Geometry: final body of the model. Coordinates: model frame, mm. A direction names the side the tool comes from. Round coordinates to 2 decimals unless told otherwise and drop trailing zeros. Order: outer loops, then holes, each group sorted by start corner. A loop starts at its lowest first (then second) coordinate and runs counter-clockwise, first axis right, second up. Notation, with made-up numbers: M -15,15 L 22,15 A25 cw 22,38 Z; hole C 71,34 d1. An arc over 180 degrees is marked long. Put each result on its own line as item: value. Start each with the question number.
1) Section D-D, the plane x = 3.5. Return loops of the section in (y, z), then the cut area to 3 significant figures.
2) Section B-B, the plane z = 0. Return loops of the section in (x, y), then the cut area to 3 significant figures.
3) Access query for faces 1 (the flat face through (-6.467, 15.21, 4.441)), 2 (the flat face through (6, 15, -10.95)), 3 (the flat face through (0, 15, -9)), 4 (the flat face through (9.5, 8, 0)), 5 (the cylindrical face through (-2.62, 14.79, 5.34)). Directions: +Z, -Z, +X, -X, +Y, -Y. A direction counts if a zero-diameter tool reaches every point of the face in a straight line with its end or side. Return the directions, or none.
4) Section A-A, the plane x = -2.5. Return loops of the section in (y, z), then the cut area to 3 significant figures.
5) First-contact query: P1, Ø3, axis at x = -4.5, y = 19.5, coming from the -Z side; P2, Ø9, axis at y = 22, z = 0, coming from the +X side; P3, Ø3, axis at x = -2, y = 21.5, coming from the -Z side. Flat tips, straight axial feed; report the tip coordinate or a pass-through.
6) Material intervals for probe 1 along Y at (x, z) = (10.4, 0); probe 2 along Z at (x, y) = (10.85, 8); probe 3 along X at (y, z) = (25.25, 4.5), sorted ascending. Write a range as [from, to].
7) Draft query along Z for faces 6 (the flat face through (0, 15, 9)), 7 (the flat face through (-6.467, 15.21, -4.441)), 8 (the cylindrical face through (-2.7, 14.8, -5.3)). Return one class per face: pulls with the +Z half, pulls with the -Z half, needs draft (parallel to the pull), parting line crosses it, or undercut.
Autodesk Inventor part; units mm, degrees
ref_plane "YZ Plane" through (0, 0, 0) normal (1, 0, 0) x (0, 1, 0)
ref_plane "XZ Plane" through (0, 0, 0) normal (0, 1, 0) x (-1, 0, 0)
ref_plane "XY Plane" through (0, 0, 0) normal (0, 0, 1) x (1, 0, 0)
sketch "Эскиз1" plane through (0, 0, 0) normal (0, 1, 0) x (-1, 0, 0)
  circle A0 centre (0, 0) radius 5.95
  circle A1 centre (0, 0) radius 6.95
  line L0 (0, 0) -> (5.546, 4.1887)
  line L1 (0, 0) -> (5.546, -4.1887)
  point P0 (4.748, -3.586)
  point P1 (4.748, 3.586)
  dimension "d0" = 11.9
  dimension "d1" = 13.9
extrude "Выдавливание1" add sketch "Эскиз1" along normal blind 30 contours A0 L1 A1 L0 picked at (4.878, 4.401)
sketch "Эскиз2" plane through (0, 30, 0) normal (0, 1, 0) x (1, 0, 0)
  arc A0 (-4.748, -3.586) -> (-5.6407, -3.0561) centre (-7.4493, -7.1199) ccw
  arc A1 (-5.6407, -3.0561) -> (-6.7976, -4.8618) centre (-6.075, -4.0513) ccw
  line L0 (-6.7976, -4.8618) -> (-6.1263, -4.0074)
  arc A2 (-5.5474, -4.1741) -> (-6.1263, -4.0074) centre (-5.9157, -4.3645) ccw
  line L1 (-4.748, -3.586) -> (-5.546, -4.1887)
  line L2 (-5.546, -4.1887) -> (-4.748, -3.586)
  line L3 (-5.546, -4.1887) -> (-5.5474, -4.1741)
  line L4 (-0.0151, 0) -> (-3.489, 0)
  arc A3 (-5.6407, 3.0561) -> (-4.748, 3.586) centre (-7.4493, 7.1199) ccw
  arc A4 (-6.1263, 4.0074) -> (-5.5474, 4.1741) centre (-5.9157, 4.3645) ccw
  line L5 (-4.748, 3.586) -> (-5.546, 4.1887)
  line L6 (-5.546, 4.1887) -> (-4.748, 3.586)
  line L7 (-5.546, 4.1887) -> (-5.5474, 4.1741)
  arc A5 (-6.7976, 4.8618) -> (-5.6407, 3.0561) centre (-6.075, 4.0513) ccw
  line L8 (-6.7976, 4.8618) -> (-6.1263, 4.0074)
  point P0 (-4.748, 3.586)
  point P1 (-5.546, -4.1887)
  point P2 (-5.3694, -4.0591)
  point P3 (-5.3694, 4.0591)
  dimension "d25" = 1.0859
sketch "Эскиз3" plane through (0, 30, 0) normal (0, 1, 0) x (1, 0, 0)
  arc A0 (-5.546, -4.1887) -> (-5.546, 4.1887) centre (0, 0) ccw
  line L0 (11.5, -6.95) -> (11.5, 6.95)
  arc A1 (-4.748, -3.586) -> (-4.748, 3.586) centre (0, 0) ccw
  line L1 (0, -6.95) -> (0, -5.95)
  line L2 (0, 5.95) -> (0, 6.95)
  line L3 (11.5, 6.95) -> (11.5, 10.95)
  line L4 (11.5, -6.95) -> (11.5, -10.95)
  line L5 (0, 2.45) -> (0, 6.95)
  line L6 (11.5, -10.95) -> (0, -10.95)
  line L7 (0, -10.95) -> (0, -6.95)
  line L8 (11.5, 10.95) -> (0, 10.95)
  line L9 (0, 10.95) -> (0, 6.95)
  arc A2 (0, -5.95) -> (0, 5.95) centre (0, 0) ccw
  dimension "d13" = 4
  dimension "d14" = 4
  dimension "d22" = 21.9
  dimension "d23" = 5
extrude "Выдавливание3" add sketch "Эскиз3" against normal blind 30
ref_plane "РабПлоскость1" through (11.5, 20, 4.95) normal (1, 0, 0) x (0, 0, -1)
sketch "Эскиз4" plane through (11.5, 20, 4.95) normal (1, 0, 0) x (0, 0, -1)
  line L0 (4.95, -20) -> (4.95, 10)
  line L1 (1, 10) -> (8.9, 10)
  circle A0 centre (4.95, -12) radius 5
  line L2 (14.4, -20) -> (-4.5, -20)
  circle A1 centre (4.95, 2) radius 5
  line L3 (-4.5, 10) -> (14.4, 10)
  point P0 (7.3306, 10)
  point P1 (2.5694, 10)
  point P2 (4.95, 10)
  dimension "d15" = 10
  dimension "d16" = 8
  dimension "d17" = 10
  dimension "d18" = 8
extrude "Выдавливание4" cut sketch "Эскиз4" against normal blind 2
extrude "Выдавливание5" add sketch "Эскиз2" against normal blind 30
sketch "Эскиз5" plane through (0, 30, 0) normal (0, 1, 0) x (1, 0, 0)
  arc A0 (0, 6.95) -> (-5.546, 4.1887) centre (0, 0) ccw
  line L0 (-5.546, 4.1887) -> (-5.5474, 4.1741)
  arc A1 (-6.1263, 4.0074) -> (-5.5474, 4.1741) centre (-5.9157, 4.3645) ccw
  line L1 (-6.1263, 4.0074) -> (-6.7976, 4.8618)
  arc A2 (-6.7976, 4.8618) -> (-5.6407, 3.0561) centre (-6.075, 4.0513) ccw
  arc A3 (-5.6407, 3.0561) -> (-4.748, 3.586) centre (-7.4493, 7.1199) ccw
  arc A4 (-4.748, -3.586) -> (-4.748, 3.586) centre (0, 0) ccw
  arc A5 (-4.748, -3.586) -> (-5.6407, -3.0561) centre (-7.4493, -7.1199) ccw
  arc A6 (-5.6407, -3.0561) -> (-6.7976, -4.8618) centre (-6.075, -4.0513) ccw
  line L2 (-6.7976, -4.8618) -> (-6.1263, -4.0074)
  arc A7 (-5.5474, -4.1741) -> (-6.1263, -4.0074) centre (-5.9157, -4.3645) ccw
  line L3 (-5.5474, -4.1741) -> (-5.546, -4.1887)
  arc A8 (-5.546, -4.1887) -> (0, -6.95) centre (0, 0) ccw
  line L4 (0, -6.95) -> (0, -10.95)
  line L5 (0, -10.95) -> (11.5, -10.95)
  line L6 (11.5, -10.95) -> (11.5, 10.95)
  line L7 (11.5, 10.95) -> (0, 10.95)
  line L8 (0, 10.95) -> (0, 6.95)
  line L9 (0, 5.95) -> (0, 6.95)
  line L10 (0, -5.95) -> (0, -6.95)
extrude "Выдавливание6" [suppressed]
sketch "Эскиз6" plane through (11.5, 30, 10.95) normal (1, 0, 0) x (0, 0, -1)
  arc A0 (15.95, -22) -> (15.95, -22) centre (10.95, -22) ccw
  arc A1 (15.95, -8) -> (15.95, -8) centre (10.95, -8) ccw
  point P0 (10.95, -30)
extrude "Выдавливание7" [suppressed]
properties part number "крепление маркера 12мм"
Result sheet:
1. outline: M 0,-10.95 L 30,-10.95 L 30,-4.81 L 0,-4.81 Z; M 0,4.81 L 30,4.81 L 30,10.95 L 0,10.95 Z
1. area: 368 mm2
2. outline: M 5.95,0 L 11.5,0 L 11.5,3 L 9.5,3 L 9.5,13 L 11.5,13 L 11.5,17 L 9.5,17 L 9.5,27 L 11.5,27 L 11.5,30 L 5.95,30 Z
2. area: 126 mm2
3. face 1: +Z, +Y, -Y
3. face 2: -Z, +X, -X, +Y, -Y
3. face 3: -Z, -X, +Y, -Y
3. face 4: +X
3. face 5: +Y, -Y
4. outline: M 0,-6.48 L 30,-6.48 L 30,-5.4 L 0,-5.4 Z; M 0,5.4 L 30,5.4 L 30,6.48 L 0,6.48 Z
4. area: 65.1 mm2
5. P1: stops at z = -6.27
5. P2: stops at x = 9.5
5. P3: stops at z = -6.93
6. probe 1: y = [0, 3], [13, 17], [27, 30]
6. probe 2: z = [-10.95, -5], [5, 10.95]
6. probe 3: x = [-7.06, -6.51], [-5.3, -3.89], [3.89, 11.5]
7. face 6: needs draft
7. face 7: pulls with the -Z half
7. face 8: undercut
